Can you work these out from the model? Positions are in its coordinate system, mm. Face numbers are marked on the shaded views. A direction names the side the tool comes from. Give positions to 0.01 mm unless a question says otherwise; leave off trailing zeros. Order: outer loops, then holes, each group sorted by start corner. A loop starts at its lowest first (then second) coordinate and runs counter-clockwise, first axis right, second up.
Item 1: I want a section at D-D, the plane y = -15.5. Write out the boundary of the cut face in (x, z).
Item 2: Which directions (+Z, -Z, +X, -X, +Y, -Y) give clear straight access to the entire face, cutting with the end or side of a thin tool? Please do the marked faces 5 and 6.
Item 3: If we mould it in two halves opening along X, with no side actions, what happens to the marked faces 1, 2, 3 and 4? For each: +X half, -X half, draft (parallel to the pull), parting line (faces both ways), or undercut.
Item 4: If I drill on line 1 along Y through (x, z) = (-15.5, 3.35); line 2 along Y through (x, z) = (0, 2.55); line 3 along Z through (x, y) = (-11, 17.75), over which ranges is the centre line in solid material (lowest first)?
Item 5: I want a section at A-A, the plane z = 10.8. Write out the boundary of the cut face in (x, y), then the cut area to 3 significant figures.
Item 6: I'm going to push flat-ended pins straight in: pin 1 Ø10 at (x, z) = (-6, 10.5) entering from -Y; pin 2 Ø2 at (x, y) = (14, 2.5) entering from +Z; pin 3 Ø1.9 at (x, y) = (-15, -16.5) entering from +Z. Where does each tip first touch, or does it pass through?
Item 7: I want a section at B-B, the plane x = -15.5. Write out the boundary of the cut face in (y, z).
Item 8: I want a section at C-C, the plane y = 15.5. Write out the boundary of the cut face in (x, z).
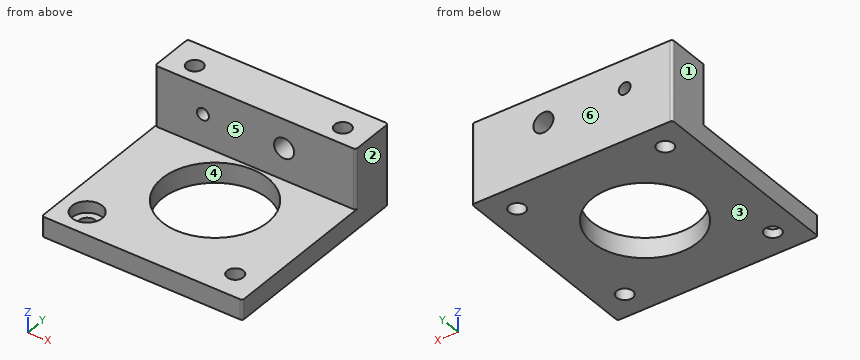
```python
from build123d import *

# Parameters (mm, degrees)
SKETCH1_W            = 42
SKETCH1_H            = 42
BOSS_EXTRUDE1_DEPTH  = 16.8
SKETCH2_W            = 42
SKETCH2_H            = 32.65
CUT_EXTRUDE1_DEPTH   = 12.6
CUT_EXTRUDE2_REACH   = 36.121
SKETCH3_R            = 11.05
M3_CLEARANCE_HOLE1_D = 3.4
SKETCH6_R            = 3.15
CUT_EXTRUDE3_DEPTH   = 2.4
M5_TAPPED_HOLE1_D    = 4.2
M3_TAPPED_HOLE1_D    = 2.5
FILLET1_R            = 0.5


with BuildPart() as part:
    # Sketch1 → Boss-Extrude1 (new body)
    with BuildSketch(Plane.XY):
        Rectangle(SKETCH1_W, SKETCH1_H)
    extrude(amount=BOSS_EXTRUDE1_DEPTH)

    # Sketch2 → Cut-Extrude1 (cut)
    with BuildSketch(Plane.XY.offset(16.8)):
        with Locations((0, -4.675)):
            Rectangle(SKETCH2_W, SKETCH2_H)
    extrude(amount=-CUT_EXTRUDE1_DEPTH, mode=Mode.SUBTRACT)

    # Sketch3 → Cut-Extrude2 (cut, up to next)
    with BuildSketch(Plane(origin=(0, 0, 0), x_dir=(-1, 0, 0), z_dir=(0, 0, -1)), mode=Mode.PRIVATE) as cut_extrude2_sk1:
        Circle(SKETCH3_R)
    cut_extrude2_tool1 = extrude(cut_extrude2_sk1.sketch, amount=-CUT_EXTRUDE2_REACH, mode=Mode.PRIVATE) & part.part
    add(cut_extrude2_tool1.solids().sort_by_distance((0, 0, 0))[0], mode=Mode.SUBTRACT)

    # M3 Clearance Hole1 (through all)
    with Locations(Plane.XY.offset(16.8)):
        with Locations((15.5, 15.5), (-15.5, 15.5), (-15.5, -15.5), (15.5, -15.5)):
            Hole(M3_CLEARANCE_HOLE1_D / 2)

    # Sketch6 → Cut-Extrude3 (cut)
    with BuildSketch(Plane.XY.offset(4.2)):
        with Locations((-15.5, -15.5)):
            Circle(SKETCH6_R)
    extrude(amount=-CUT_EXTRUDE3_DEPTH, mode=Mode.SUBTRACT)

    # M5 Tapped Hole1 (through all)
    with Locations(Plane(origin=(0, 21, 0), x_dir=(1, 0, 0), z_dir=(0, 1, 0))):
        with Locations((6, -10.8)):
            Hole(M5_TAPPED_HOLE1_D / 2)

    # M3 Tapped Hole1 (through all)
    with Locations(Plane(origin=(0, 21, 0), x_dir=(1, 0, 0), z_dir=(0, 1, 0))):
        with Locations((-11, -10.8)):
            Hole(M3_TAPPED_HOLE1_D / 2)

    # Fillet1
    fillet1_edges = [part.edges().sort_by_distance(p)[0] for p in [
        (21, -21, 2.1),
        (-21, -21, 2.1),
        (-21, 11.65, 10.5),
        (21, 11.65, 10.5),
        (-21, 21, 8.4),
        (21, 21, 8.4),
    ]]
    fillet(fillet1_edges, radius=FILLET1_R)


solid = part.part
```
Results list:
1. outline: (-21, 0) - (-17.2, 0) - (-17.2, 1.8) - (-18.65, 1.8) - (-18.65, 4.2) - (-21, 4.2) - close; (-13.8, 0) - (13.8, 0) - (13.8, 4.2) - (-12.35, 4.2) - (-12.35, 1.8) - (-13.8, 1.8) - close; (17.2, 0) - (21, 0) - (21, 4.2) - (17.2, 4.2) - close
2. face 5: +Z, +X, -X, -Y
2. face 6: +Z, -Z, +X, -X, +Y
3. face 1: -X half
3. face 2: +X half
3. face 3: draft
3. face 4: undercut
4. line 1: y = -21 to -18.65, -12.35 to 13.8, 17.2 to 21
4. line 2: y = -21 to -11.05, 11.05 to 21
4. line 3: z = 0 to 9.55, 12.05 to 16.8
5. outline: (-21, 12.15) arc R0.5 ccw to (-20.5, 11.65) - (-12.25, 11.65) - (-12.25, 21) - (-20.5, 21) arc R0.5 ccw to (-21, 20.5) - close; (-9.75, 11.65) - (3.9, 11.65) - (3.9, 21) - (-9.75, 21) - close; (8.1, 11.65) - (20.5, 11.65) arc R0.5 ccw to (21, 12.15) - (21, 20.5) arc R0.5 ccw to (20.5, 21) - (8.1, 21) - close; hole circle Ø3.4 at (-15.5, 15.5); hole circle Ø3.4 at (15.5, 15.5)
5. area: 312 mm2
6. pin 1: stops at y = 11.65
6. pin 2: stops at z = 4.2
6. pin 3: stops at z = 1.8
7. outline: (-21, 0) - (-17.2, 0) - (-17.2, 1.8) - (-18.65, 1.8) - (-18.65, 4.2) - (-21, 4.2) - close; (-13.8, 0) - (13.8, 0) - (13.8, 16.8) - (11.65, 16.8) - (11.65, 4.2) - (-12.35, 4.2) - (-12.35, 1.8) - (-13.8, 1.8) - close; (17.2, 0) - (21, 0) - (21, 16.8) - (17.2, 16.8) - close
8. outline: (-21, 0) - (-17.2, 0) - (-17.2, 16.8) - (-21, 16.8) - close; (-13.8, 0) - (13.8, 0) - (13.8, 16.8) - (-13.8, 16.8) - close; (17.2, 0) - (21, 0) - (21, 16.8) - (17.2, 16.8) - close; hole circle Ø2.5 at (-11, 10.8); hole circle Ø4.2 at (6, 10.8)
